For this review, use the dimensioned drawing (mm, ordinates from the lowest corner) and the shaded views. A direction names the side the tool comes from. Coordinates: 2 decimals unless noted, no trailing zeros. Order: outer loops, then holes, each group sorted by start corner. A loop starts at its lowest first (then second) coordinate and runs counter-clockwise, first axis right, second up. Notation, with made-up numbers: (2.25, 86.25) -> (16.25, 86.25) arc R5 cw to (16.25, 92.25) -> close; hole circle Ø2 at (23.25, -34.5). An arc over 180 degrees is marked (long way). Use one line per item in the form item = value. Start each with the question number.
(1) For the marked faces 4 and 5, list the 3-axis set-ups (+Z, -Z, +X, -X, +Y, -Y) from which the entire face can be reached by the end or side of a thin tool; tool diameter is ignored.
(2) Take a section at C-C (x = 2.2). State the section outline as (y, z) points, then the cut area to 3 significant figures.
(3) Take a section at A-A (x = 3.75). State the section outline as (y, z) points.
(4) Mouldability with a two-part tool opening along Y and no side actions: class the marked faces 1, 2 and 3 as +Y half, -Y half, draft (parallel to the pull), parting line (faces both ways), or undercut.
(5) Insertion check: pin 1 Ø4.5 at (y, z) = (4.5, 7) entering from -X; pin 2 Ø3 at (y, z) = (12.5, 4) entering from -X; pin 3 Ø1.8 at (x, z) = (2.2, 1.6) entering from -Y. Each pin has a flat end and moves straight along its axis. Give the tip position at first contact, or say it passes through.
(6) Take a section at B-B (z = 1.6). State the section outline as (x, y) points.
(7) Take a section at D-D (y = 15). State the section outline as (x, z) points.
(8) Wall thickness on line 1 along Y through (x, z) = (7.25, 5.75); line 2 along Y through (x, z) = (3.25, 9.25); line 3 along Z through (x, y) = (2.2, 0.5): over which ranges is each line inside the solid? List them lowest first.
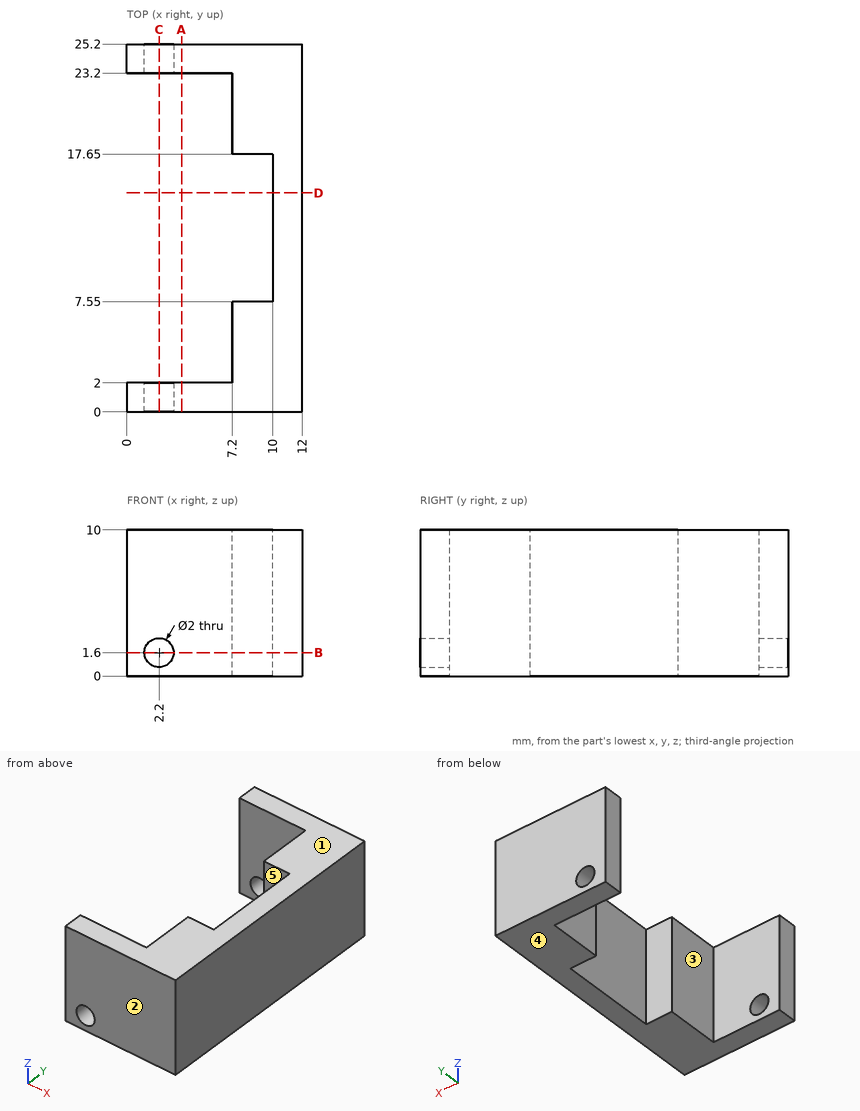
Findings:
q1.face_4 = -Z, +X, -X, +Y, -Y
q1.face_5 = +Z, -Z, -X
q2.outline = (0, 0) -> (2, 0) -> (2, 0.6) -> (0, 0.6) -> close; (0, 2.6) -> (2, 2.6) -> (2, 10) -> (0, 10) -> close; (23.2, 0) -> (25.2, 0) -> (25.2, 0.6) -> (23.2, 0.6) -> close; (23.2, 2.6) -> (25.2, 2.6) -> (25.2, 10) -> (23.2, 10) -> close
q2.area = 32.0 mm²
q3.outline = (0, 0) -> (2, 0) -> (2, 10) -> (0, 10) -> close; (23.2, 0) -> (25.2, 0) -> (25.2, 10) -> (23.2, 10) -> close
q4.face_1 = draft
q4.face_2 = -Y half
q4.face_3 = undercut
q5.pin_1 = 7.2
q5.pin_2 = 10
q5.pin_3 = through
q6.outline = (0, 0) -> (1.2, 0) -> (1.2, 2) -> (0, 2) -> close; (0, 23.2) -> (1.2, 23.2) -> (1.2, 25.2) -> (0, 25.2) -> close; (3.2, 0) -> (12, 0) -> (12, 25.2) -> (3.2, 25.2) -> (3.2, 23.2) -> (7.2, 23.2) -> (7.2, 17.65) -> (10, 17.65) -> (10, 7.55) -> (7.2, 7.55) -> (7.2, 2) -> (3.2, 2) -> close
q7.outline = (10, 0) -> (12, 0) -> (12, 10) -> (10, 10) -> close
q8.line_1 = 0 to 7.55, 17.65 to 25.2
q8.line_2 = 0 to 2, 23.2 to 25.2
q8.line_3 = 0 to 0.6, 2.6 to 10
